Verification items for this drawing (mm, ordinates from the low corner). A direction names the side the tool comes from. Round coordinates to 2 decimals unless told otherwise and drop trailing zeros. Order: outer loops, then holes, each group sorted by start corner. A loop starts at its lowest first (then second) coordinate and runs counter-clockwise, first axis right, second up. Notation, with made-up numbers: (30.25, 81) -> (40.25, 81) arc R29 ccw to (40.25, 106) -> close; hole circle Ø2 at (1, 69.5). An arc over 180 degrees is marked (long way). Put each result on its own line as item: value.
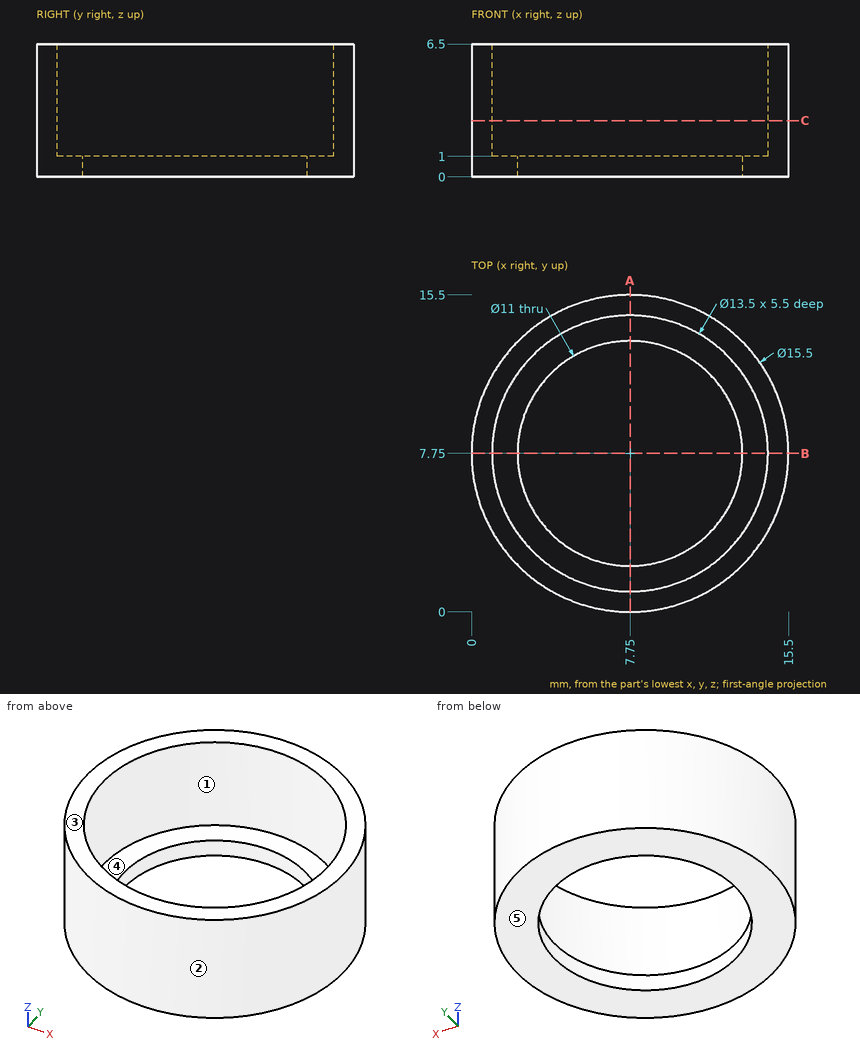
Item 1: Section check C-C on z = 2.75. Record the boundary of the cut face in (x, y).
Check sheet entries:
outline: circle Ø15.5 at (7.75, 7.75); hole circle Ø13.5 at (7.75, 7.75)
Item 2: Gauge pin test, flat ends, axial feed: pin 1 Ø3 at (y, z) = (6, 4) entering from +X; pin 2 Ø2 at (x, z) = (12, 2.5) entering from -Y. Record the tip position at first contact, or that the pin passes through.
Check sheet entries:
pin 1: stops at x = 15.5
pin 2: stops at y = 0.71
Item 3: Release check for a two-part mould opening along X. For the marked faces 1, 2 and 3 record: +X half, -X half, draft (parallel to the pull), parting line (faces both ways), or undercut.
Check sheet entries:
face 1: undercut
face 2: parting line
face 3: draft
Item 4: Section check A-A on x = 7.75. Record the boundary of the cut face in (y, z).
Check sheet entries:
outline: (0, 0) -> (2.25, 0) -> (2.25, 1) -> (1, 1) -> (1, 6.5) -> (0, 6.5) -> close; (13.25, 0) -> (15.5, 0) -> (15.5, 6.5) -> (14.5, 6.5) -> (14.5, 1) -> (13.25, 1) -> close
Item 5: Tool access check on the marked faces 4 and 5. Record the directions out of +Z, -Z, +X, -X, +Y, -Y that give a thin tool (end or side, any length) a straight path to the whole face; none if there is none.
Check sheet entries:
face 4: +Z
face 5: -Z, +X, -X, +Y, -Y
Item 6: Material ranges on L1, parallel to Y at x = 8, z = 6.25; L2, parallel to Y at x = 7.75, z = 0.4; L3, parallel to X at y = 1.5, z = 5.25, recorded low to high. Write a range as [from, to].
Check sheet entries:
L1: y = [0, 1], [14.5, 15.5]
L2: y = [0, 2.25], [13.25, 15.5]
L3: x = [3.17, 5.2], [10.3, 12.33]
